Work out the finished part from the listing and answer in its coordinate system (mm). Face numbers are marked on the shaded views. A direction names the side the tool comes from. Coordinates: 2 decimals unless noted, no trailing zeros. Order: outer loops, then holes, each group sorted by start corner. A loop starts at its lowest first (then second) coordinate and runs counter-clockwise, first axis right, second up. Notation, with made-up numbers: (16.25, 84) -> (74.25, 84) arc R20 cw to (74.25, 123) -> close; hole circle Ø6 at (24.5, -0.75). An arc over 180 degrees is marked (long way). Answer as CSV lines item,"result". Start each with the question number.
Item 1: Each of these flat-tipped pins is pushed along its axis until it touches: pin 1 Ø3 at (y, z) = (-6.5, 0) entering from -X; pin 2 Ø8 at (x, y) = (0.5, -17) entering from -Z; pin 3 Ø9 at (x, y) = (-15.5, -15) entering from +Z. Where does it stop, or does it pass through?
Item 2: Section C-C (y = -11.5) is taken. Write down the section's boundary in (x, z), then the cut area to 3 significant figures.
Item 3: Section A-A (z = -3) is taken. Write down the section's boundary in (x, y).
Item 4: Section D-D (z = 0) is taken. Write down the section's boundary in (x, y), then the cut area to 3 significant figures.
Item 5: Section B-B (x = -14.5) is taken. Write down the section's boundary in (y, z).
Item 6: Which of the six approach directions +Z, -Z, +X, -X, +Y, -Y give full straight-line access (tool end or side, diameter ignored) to the marked faces 4, 5 and 6?
Item 7: Straight lines are drawn through the part: L1, parallel to X at y = -16.25, z = -1.5; L2, parallel to X at y = -10, z = -2.5; L3, parallel to Y at x = -14.5, z = -3.45. For each, find the intervals that lie inside material, in ascending order.
Item 8: For a pull along X with two mould halves and no side action, classify the marked faces 1, 2 and 3 as pulls with the +X half, pulls with the -X half, needs draft (parallel to the pull), parting line crosses it, or undercut.
```python
from build123d import *

# Parameters (mm, degrees)
F1_DEPTH = 23
F2_R     = 2
F3_DEPTH = 25


with BuildPart() as f1:
    # F0 (on Front) → F1 (new body)
    with BuildSketch(Plane.XZ):
        Polygon((20, -6), (20, -2), (9, -2), (9, 6), (8, 6), (-8, 6), (-9, 6), (-9, -2), (-20, -2), (-20, -6), (-6, -6), (-6, 0), (-6, 2), (6, 2), (6, 0), (6, -6), align=None)
    extrude(amount=F1_DEPTH)

    # F2 (on Top) → F3 (cut)
    with BuildSketch(Plane.XY):
        with Locations((-14.5, -11.5)):
            Circle(F2_R)
        with Locations((14.5, -11.5)):
            Circle(F2_R)
    extrude(amount=-F3_DEPTH, mode=Mode.SUBTRACT)


solid = f1.part
```
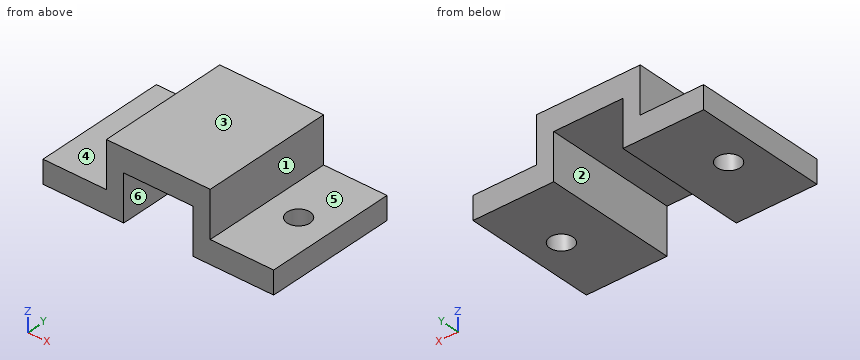
Checked values:
1,pin 1,"stops at x = -9"
1,pin 2,"stops at z = 2"
1,pin 3,"stops at z = -2"
2,outline,"(-20, -6) -> (-16.5, -6) -> (-16.5, -2) -> (-20, -2) -> close; (-12.5, -6) -> (-6, -6) -> (-6, 2) -> (6, 2) -> (6, -6) -> (12.5, -6) -> (12.5, -2) -> (9, -2) -> (9, 6) -> (-9, 6) -> (-9, -2) -> (-12.5, -2) -> close; (16.5, -6) -> (20, -6) -> (20, -2) -> (16.5, -2) -> close"
2,area,"176 mm^2"
3,outline,"(-20, -23) -> (-6, -23) -> (-6, 0) -> (-20, 0) -> close; (6, -23) -> (20, -23) -> (20, 0) -> (6, 0) -> close; hole circle Ø4 at (-14.5, -11.5); hole circle Ø4 at (14.5, -11.5)"
4,outline,"(-9, -23) -> (-6, -23) -> (-6, 0) -> (-9, 0) -> close; (6, -23) -> (9, -23) -> (9, 0) -> (6, 0) -> close"
4,area,"138 mm^2"
5,outline,"(-23, -6) -> (-13.5, -6) -> (-13.5, -2) -> (-23, -2) -> close; (-9.5, -6) -> (0, -6) -> (0, -2) -> (-9.5, -2) -> close"
6,face 4,"+Z, -X, +Y, -Y"
6,face 5,"+Z, +X, +Y, -Y"
6,face 6,"-Z, +Y, -Y"
7,L1,"x = -9 to -6, 6 to 9"
7,L2,"x = -20 to -15.82, -13.18 to -6, 6 to 13.18, 15.82 to 20"
7,L3,"y = -23 to -13.5, -9.5 to 0"
8,face 1,"pulls with the +X half"
8,face 2,"undercut"
8,face 3,"needs draft"
